Could you check a few things on this model? Use its own coordinates, in mm. Face numbers are marked on the shaded views. Give positions to 0.01 mm unless a question says otherwise; leave off trailing zeros. Write each loop counter-clockwise with the first axis right and the second up, starting at its lowest first coordinate (ties: lowest second). Pieces come first, ordered by that corner, then holes. Notation, with made-up numbers: M 71.5,16.25 L 119.5,16.25 A26 cw 119.5,38.25 Z; hole C -31.75,41.25 d8. An arc over 180 degrees is marked long. Answer as a JSON object with one key per item and string values. Group by question number.
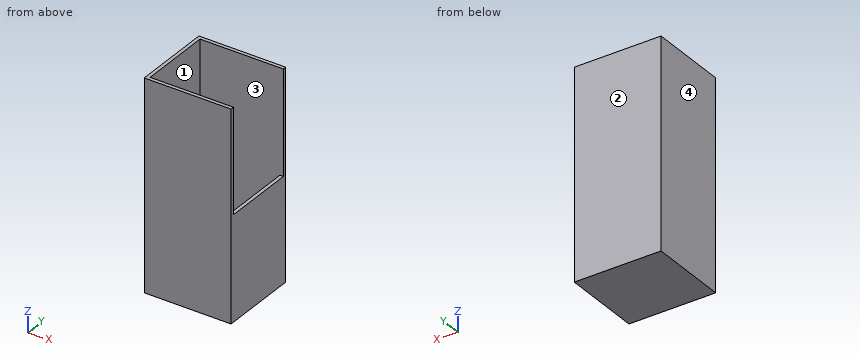
```python
from build123d import *

# Parameters (mm, degrees)
F0_W     = 63.5
F0_H     = 152.4
F1_DEPTH = 58.42
F2_T     = -2.54
F3_W     = 53.34
F3_H     = 76.2
F4_DEPTH = 25.4


with BuildPart() as f1:
    # F0 (on Front) → F1 (new body)
    with BuildSketch(Plane.XZ):
        with Locations((0, -10.713868)):
            Rectangle(F0_W, F0_H)
    extrude(amount=-F1_DEPTH)

    # F2
    f2_openings = [f1.faces().sort_by_distance(p)[0] for p in [
        (0, 29.21, 65.486132),
    ]]
    offset(amount=F2_T, openings=f2_openings)

    # F3 (on face) → F4 (cut)
    with BuildSketch(Plane.YZ.offset(31.75)):
        with Locations((29.21, 27.386132)):
            Rectangle(F3_W, F3_H)
    extrude(amount=-F4_DEPTH, mode=Mode.SUBTRACT)


solid = f1.part
```
1) I'm going to push flat-ended pins straight in: pin 1 (4 mm diameter, centred on x = 6.5, y = 49.5, fed in from +Z); pin 2 (3 mm diameter, centred on x = 30, y = 22.5, fed in from +Z). Where does each tip first touch, or does it pass through?
2) We'd pull the mould along X, two halves only. Please class the marked faces 1, 2, 3 and 4: released by +X, released by -X, zero draft, split by the parting line, or undercut.
3) Please list where these lines run through material, in increasing order: line 1 along Y through (x, z) = (3, 32.5); line 2 along X through (y, z) = (27.5, -14.5); line 3 along Z through (x, y) = (-10, 29.5). Write a range as from..to.
4) If we section it at A-A, the plane z = -37.5: List the corners of the cut face in (x, y) for me.
5) If we section it at B-B, the plane x = -17.5: List the corners of the cut face in (y, z) for me.
6) If we section it at C-C, the plane y = 21: List the corners of the cut face in (x, z) for me, plus the area to 3 significant figures.
Taken from the geometry:
{
 "1": {"pin 1": "z = -84.37", "pin 2": "z = -10.71"},
 "2": {"face 1": "undercut", "face 2": "zero draft", "face 3": "undercut", "face 4": "released by -X"},
 "3": {"line 1": "0..2.54, 55.88..58.42", "line 2": "-31.75..-29.21, 29.21..31.75", "line 3": "-86.91..-84.37"},
 "4": {"outline": "M -31.75,0 L 31.75,0 L 31.75,58.42 L -31.75,58.42 Z; hole M -29.21,2.54 L 29.21,2.54 L 29.21,55.88 L -29.21,55.88 Z"},
 "5": {"outline": "M 0,-86.91 L 58.42,-86.91 L 58.42,65.49 L 55.88,65.49 L 55.88,-84.37 L 2.54,-84.37 L 2.54,65.49 L 0,65.49 Z"},
 "6": {"outline": "M -31.75,-86.91 L 31.75,-86.91 L 31.75,-10.71 L 29.21,-10.71 L 29.21,-84.37 L -29.21,-84.37 L -29.21,65.49 L -31.75,65.49 Z", "area": "729 mm²"}
}
